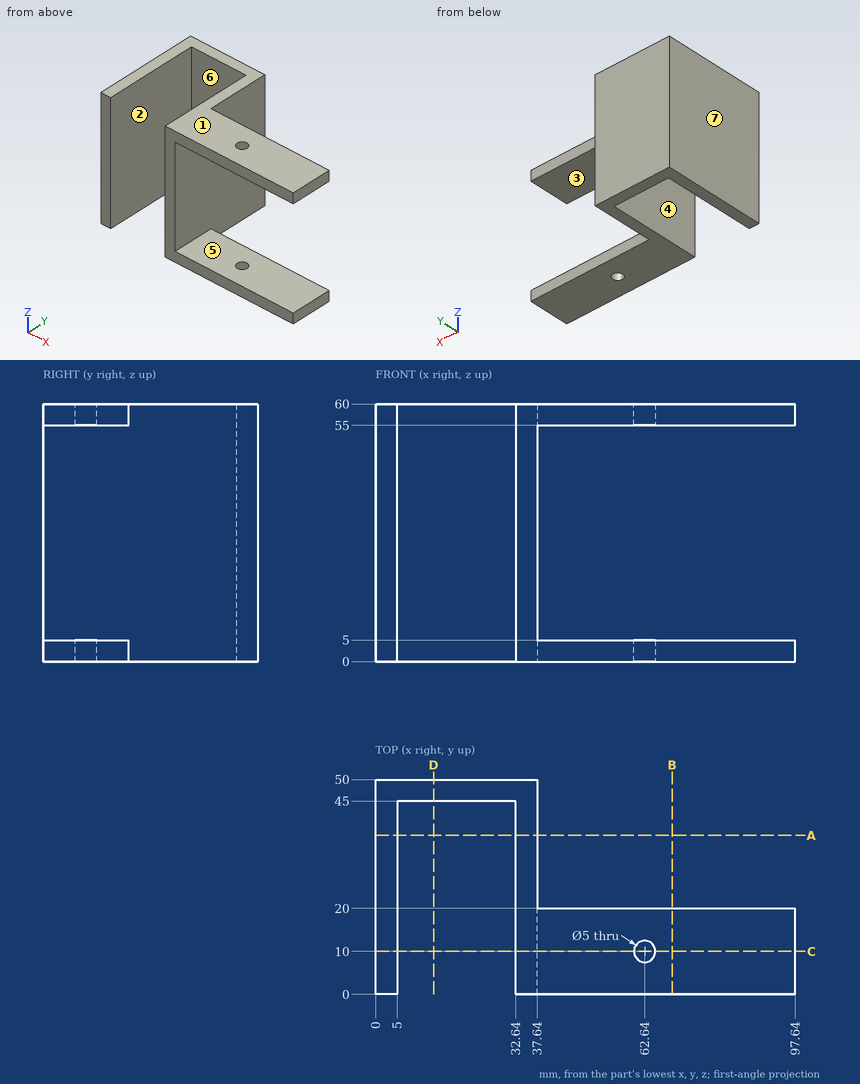
Verification items for this drawing (mm, ordinates from the low corner). A direction names the side the tool comes from. Coordinates: 2 decimals unless noted, no trailing zeros. Loops run counter-clockwise (first coordinate to the right, second up) from the corner with the lowest first, then second, coordinate; pieces in that order, holes last. Notation, with made-up numbers: (8.25, 17) -> (40.25, 17) arc R15 ccw to (40.25, 35) -> close; hole circle Ø4 at (83, 0.5). An arc over 180 degrees is marked (long way). Answer in a Markdown table with one row per item. Add a question column.
1. Material ranges on probe 1 along X at (y, z) = (7, 33); probe 2 along X at (y, z) = (6, 4.5); probe 3 along Z at (x, y) = (52.5, 10), recorded low to high. Write a range as [from, to].
2. Section check D-D, the plane x = 13.5. Enter the section's corners in (y, z), then the cut area to 3 significant figures.
3. Draft check along X on the marked faces 4, 5, 6 and 7. Enter one of: +X half, -X half, draft (parallel to the pull), parting line (faces both ways), or undercut.
4. Section check C-C, the plane y = 10. Enter the section's corners in (x, z), then the cut area to 3 significant figures.
5. Section check A-A, the plane y = 37. Enter the section's corners in (x, z), then the cut area to 3 significant figures.
6. Depth check by flat-ended pin: P1, Ø1.5, axis at x = 75.5, z = 58.5, coming from the +Y side; P2, Ø3, axis at y = 23.5, z = 40.5, coming from the +X side; P3, Ø22, axis at x = 16.5, z = 24.5, coming from the -Y side. Enter the tip coordinate at first touch or a pass-through.
7. Section check B-B, the plane x = 69. Enter the section's corners in (y, z).
8. Access from +Z, -Z, +X, -X, +Y, -Y to the whole of each face (thin tool, end or side, straight path). Record for the marked faces 1, 2 and 3.
Derived:
| question | item | result |
|---|---|---|
| 1 | probe 1 | x = [0, 5], [32.64, 37.64] |
| 1 | probe 2 | x = [0, 5], [32.64, 97.64] |
| 1 | probe 3 | z = [0, 5], [55, 60] |
| 2 | outline | (45, 0) -> (50, 0) -> (50, 60) -> (45, 60) -> close |
| 2 | area | 300 mm² |
| 3 | face 4 | undercut |
| 3 | face 5 | draft |
| 3 | face 6 | undercut |
| 3 | face 7 | -X half |
| 4 | outline | (0, 0) -> (5, 0) -> (5, 60) -> (0, 60) -> close; (32.64, 0) -> (60.14, 0) -> (60.14, 5) -> (37.64, 5) -> (37.64, 55) -> (60.14, 55) -> (60.14, 60) -> (32.64, 60) -> close; (65.14, 0) -> (97.64, 0) -> (97.64, 5) -> (65.14, 5) -> close; (65.14, 55) -> (97.64, 55) -> (97.64, 60) -> (65.14, 60) -> close |
| 4 | area | 1,150 mm² |
| 5 | outline | (0, 0) -> (5, 0) -> (5, 60) -> (0, 60) -> close; (32.64, 0) -> (37.64, 0) -> (37.64, 60) -> (32.64, 60) -> close |
| 5 | area | 600 mm² |
| 6 | P1 | stops at y = 20 |
| 6 | P2 | stops at x = 37.64 |
| 6 | P3 | stops at y = 45 |
| 7 | outline | (0, 0) -> (20, 0) -> (20, 5) -> (0, 5) -> close; (0, 55) -> (20, 55) -> (20, 60) -> (0, 60) -> close |
| 8 | face 1 | +Z, +X, -X, +Y, -Y |
| 8 | face 2 | +Z, -Z, -Y |
| 8 | face 3 | +X, +Y, -Y |
